Geometry: see drawing. Coordinates: mm, zero at the bounding-box minimum. A direction names the side the tool comes from. Coordinates: 2 decimals unless noted, no trailing zeros. Loops run counter-clockwise (first coordinate to the right, second up) from the corner with the lowest first, then second, coordinate; pieces in that order, holes last. Notation, with made-up numbers: (-10.75, 4) -> (-6.75, 4) arc R20 cw to (-6.75, 31) -> close; hole circle Ø4 at (-25.75, 27). An arc over 180 degrees is marked (long way). One line per question, with ' | ' between items. Start each with the question number.
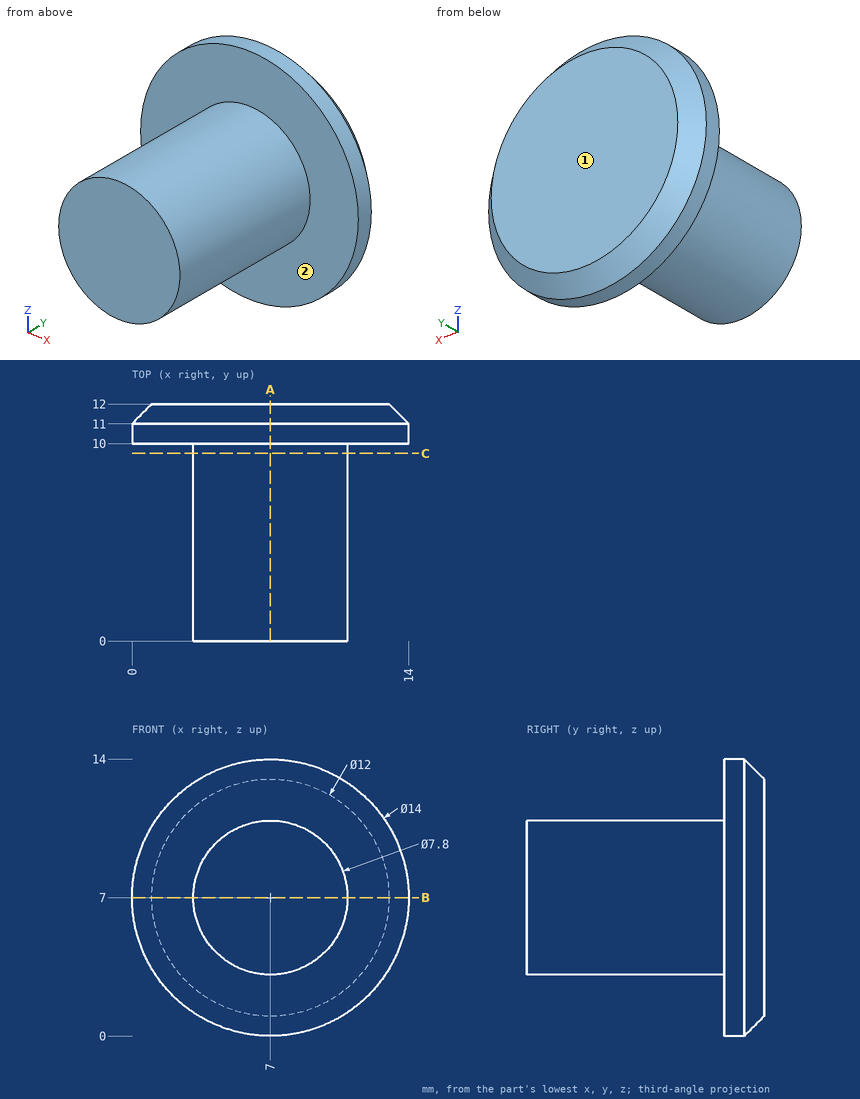
(1) Contact query for flat-ended pins moving along their axis: pin 1 Ø7 at (x, z) = (4.5, 8) entering from -Y; pin 2 Ø4 at (x, y) = (7, 7) entering from -Z; pin 3 Ø1 at (x, z) = (10, 3) entering from -Y; pin 4 Ø2 at (y, z) = (3.5, 8) entering from +X. Output: stop coordinate, or through.
(2) Cut plane C-C, the plane y = 9.5. Return the cut outline in (x, z).
(3) Ray query, L1, parallel to Y at x = 11, z = 4.5; L2, parallel to Z at x = 7, y = 8.25; L3, parallel to X at y = 8, z = 8.75. Return the intervals inside material, ascending.
(4) Access query for the marked faces 1 and 2. Directions: +Z, -Z, +X, -X, +Y, -Y. A direction counts if a zero-diameter tool reaches every point of the face in a straight line with its end or side. Return the directions, or none.
(5) Cut plane B-B, the plane z = 7. Return the cut outline in (x, y).
(6) Cut plane A-A, the plane x = 7. Return the cut outline in (y, z), and give its area (3 significant figures).
Here are the results:
1) pin 1: stops at y = 0 | pin 2: stops at z = 3.1 | pin 3: stops at y = 10 | pin 4: stops at x = 10.9
2) outline: circle Ø7.8 at (7, 7)
3) L1: y = 10 to 12 | L2: z = 3.1 to 10.9 | L3: x = 3.51 to 10.49
4) face 1: +Z, -Z, +X, -X, +Y | face 2: -Y
5) outline: (0, 10) -> (3.1, 10) -> (3.1, 0) -> (10.9, 0) -> (10.9, 10) -> (14, 10) -> (14, 11) -> (13, 12) -> (1, 12) -> (0, 11) -> close
6) outline: (0, 3.1) -> (10, 3.1) -> (10, 0) -> (11, 0) -> (12, 1) -> (12, 13) -> (11, 14) -> (10, 14) -> (10, 10.9) -> (0, 10.9) -> close | area: 105 mm2
